from build123d import *

# Parameters (mm, degrees)
F0_W     = 165.1
F0_H     = 82.55
F3_DEPTH = 25.4
F1_W     = 25.4
F1_H     = 25.4
F4_DEPTH = 812.8
F2_R     = 12.7
F5_DEPTH = 1752.6


with BuildPart() as f3:
    # F0 (on Front) → F3 (new body)
    with BuildSketch(Plane.XZ):
        with Locations((-82.55, 41.275)):
            Rectangle(F0_W, F0_H)
    extrude(amount=F3_DEPTH)

    # F1 (on face) → F4 (cut)
    with BuildSketch(Plane.XZ):
        with Locations((-122.377806, 41.276296)):
            Rectangle(F1_W, F1_H)
    extrude(amount=F4_DEPTH, mode=Mode.SUBTRACT)

    # F2 (on face) → F5 (cut)
    with BuildSketch(Plane.XZ):
        with Locations((-38.1, 38.1)):
            Circle(F2_R)
    extrude(amount=F5_DEPTH, mode=Mode.SUBTRACT)


solid = f3.part
Read the model definition and answer for the solid it produces. Units are mm, in the model's axes. A direction names the side the tool comes from. Coordinates: 2 decimals unless noted, no trailing zeros. Loops run counter-clockwise (first coordinate to the right, second up) from the corner with the lowest first, then second, coordinate; pieces in that order, holes last. Notation, with made-up numbers: (1, 27) - (7, 27) arc R3 cw to (7, 32) - close; hole circle Ø10 at (86, -29.5). An arc over 180 degrees is marked (long way). Answer in a Markdown table with one row per item.
Q1. Find section A-A on z = 38.1. Write down the section's boundary in (x, y).
Here are the results:
| item | result |
|---|---|
| outline | (-165.1, -25.4) - (-135.08, -25.4) - (-135.08, 0) - (-165.1, 0) - close; (-109.68, -25.4) - (-50.8, -25.4) - (-50.8, 0) - (-109.68, 0) - close; (-25.4, -25.4) - (0, -25.4) - (0, 0) - (-25.4, 0) - close |
Q2. For faces 5 (the flat face through (-84, -25.4, 42)), 6 (the flat face through (-123, -13, 53.976)), determine the directions among +Z, -Z, +X, -X, +Y, -Y from which every point of the face is accessible in a straight line to the end or side of a thin tool.
Here are the results:
| item | result |
|---|---|
| face 5 | +Z, -Z, +X, -X, -Y |
| face 6 | +Y, -Y |
Q3. Find section C-C on y = -4. Write down the section's boundary in (x, z), plus the area to 3 significant figures.
Here are the results:
| item | result |
|---|---|
| outline | (-165.1, 0) - (0, 0) - (0, 82.55) - (-165.1, 82.55) - close; hole (-135.08, 28.58) - (-109.68, 28.58) - (-109.68, 53.98) - (-135.08, 53.98) - close; hole circle Ø25.4 at (-38.1, 38.1) |
| area | 12,500 mm^2 |
Q4. Straight lines are drawn through the part: line 1 along X through (y, z) = (-18.75, 38.1); line 2 along X through (y, z) = (-23.75, 35); line 3 along Z through (x, y) = (-38.1, -17.25). For each, find the intervals that lie inside material, in ascending order. Write a range as [from, to].
Here are the results:
| item | result |
|---|---|
| line 1 | x = [-165.1, -135.08], [-109.68, -50.8], [-25.4, 0] |
| line 2 | x = [-165.1, -135.08], [-109.68, -50.42], [-25.78, 0] |
| line 3 | z = [0, 25.4], [50.8, 82.55] |
Q5. The mould has two halves that part along Z. Classify faces 1 (the flat face through (-165.1, -13, 41)), 2 (the flat face through (-84, -13, 0)), 3 (the cylindrical face through (-39.753, -12.522, 50.692)), 4 (the flat face through (-123, -13, 28.576)): pulls with the +Z half, pulls with the -Z half, needs draft (parallel to the pull), parting line crosses it, or undercut.
Here are the results:
| item | result |
|---|---|
| face 1 | needs draft |
| face 2 | pulls with the -Z half |
| face 3 | undercut |
| face 4 | undercut |
Q6. Find section B-B on x = -38.1. Write down the section's boundary in (y, z), plus the area to 3 significant figures.
Here are the results:
| item | result |
|---|---|
| outline | (-25.4, 0) - (0, 0) - (0, 25.4) - (-25.4, 25.4) - close; (-25.4, 50.8) - (0, 50.8) - (0, 82.55) - (-25.4, 82.55) - close |
| area | 1,450 mm^2 |
